Autodesk Inventor part; units mm, degrees
ref_plane "YZ Plane" through (0, 0, 0) normal (1, 0, 0) x (0, 1, 0)
ref_plane "XZ Plane" through (0, 0, 0) normal (0, 1, 0) x (-1, 0, 0)
ref_plane "XY Plane" through (0, 0, 0) normal (0, 0, 1) x (1, 0, 0)
sketch "Skizze1" plane through (0, 0, 0) normal (0, 1, 0) x (-1, 0, 0)
  line L0 (-37, 40) -> (37, 40)
  line L1 (40, 37) -> (40, -37)
  line L2 (37, -40) -> (-37, -40)
  line L3 (-40, -37) -> (-40, 37)
  line L4 (-40, 40) -> (40, -40) construction
  line L5 (40, 40) -> (-40, -40) construction
  arc A0 (40, 37) -> (37, 40) centre (37, 37) ccw
  arc A1 (-37, 40) -> (-40, 37) centre (-37, 37) ccw
  arc A2 (-40, -37) -> (-37, -40) centre (-37, -37) ccw
  arc A3 (37, -40) -> (40, -37) centre (37, -37) ccw
  point P0 (0, 0)
  dimension "d0" = 80
  dimension "d1" = 80
  dimension "d2" = 3
  dimension "d3" = 3
  dimension "d4" = 3
  dimension "d5" = 3
extrude "Extrusion1" add sketch "Skizze1" along normal blind 12
sketch "Skizze2" plane through (0, 12, 0) normal (0, 1, 0) x (1, 0, 0)
  line L0 (-40, 37) -> (-40, -37)
  arc A0 (-40, -37) -> (-37, -40) centre (-37, -37) ccw
  line L1 (-37, -40) -> (37, -40)
  arc A1 (37, -40) -> (40, -37) centre (37, -37) ccw
  line L2 (40, -37) -> (40, 37)
  arc A2 (40, 37) -> (37, 40) centre (37, 37) ccw
  line L3 (37, 40) -> (-37, 40)
  arc A3 (-37, 40) -> (-40, 37) centre (-37, 37) ccw
  line L4 (-35, -35) -> (-35, 35) construction
  line L5 (-35, 35) -> (35, 35) construction
  line L6 (35, 35) -> (35, -28)
  line L7 (28, -35) -> (-35, -35)
  line L8 (-35, -35) -> (-40, -35)
  line L9 (35, 35) -> (35, 40)
  arc A4 (28, -35) -> (35, -28) centre (32, -32) ccw
  point P0 (0, 0)
  dimension "d8" = 5
  dimension "d21" = 10
extrude "Extrusion2" cut sketch "Skizze2" against normal blind 6 contours A3 L3 L9 L6 A4 L7 L8 L0
fillet "Rundung1" radius 2 1 edges at (-40, 9, 35)
sketch "Skizze3" plane through (0, 0, 0) normal (0, -1, 0) x (1, 0, 0)
  arc A0 (-40, -37) -> (-37, -40) centre (-37, -37) ccw
  line L0 (-37, -37) -> (0, 0) construction
  line L1 (-37, -37) -> (-29.9289, -29.9289) construction
  dimension "d13" = 10
hole "Bohrung1" at (-29.9289, 0, -29.9289) direction (0, 1, 0) diameter 2.459 end through all
sketch "Skizze4" plane through (-37, 0, 40) normal (0, 0, 1) x (1, 0, 0)
  line L0 (-3, 0) -> (0, 0)
  line L1 (74, 0) -> (0, 0)
  line L2 (74, 0) -> (77, 0)
  line L3 (-3, 2) -> (0, 2)
  line L4 (0, 2) -> (74, 2)
  line L5 (74, 2) -> (77, 2)
  line L6 (-3, 0) -> (-3, 6)
  line L7 (77, 0) -> (77, 12)
  point P0 (37, 0)
  dimension "d22" = 2
extrude "Extrusion3" cut sketch "Skizze4" against normal blind 80
properties part number "Tastplatte" material "Aluminium 6061"
Geometry: final body of the model. Coordinates: model frame, mm. A direction names the side the tool comes from. Round coordinates to 2 decimals unless told otherwise and drop trailing zeros. Order: outer loops, then holes, each group sorted by start corner. A loop starts at its lowest first (then second) coordinate and runs counter-clockwise, first axis right, second up. Notation, with made-up numbers: (44, 63.25) - (91, 63.25) arc R4 cw to (91, 70.25) - close; hole circle Ø7 at (-10, 23.25). An arc over 180 degrees is marked (long way). Write item = value, one per line. Start each with the question number.
Q1. Access query for faces 5 (the cylindrical face through (39.14, 6.93, 39.1)), 6 (the cylindrical face through (-39.43, 8.96, 35.6)). Directions: +Z, -Z, +X, -X, +Y, -Y. A direction counts if a zero-diameter tool reaches every point of the face in a straight line with its end or side. Return the directions, or none.
Q2. Cut plane C-C on x = 32. Return the cut outline in (y, z), and give its area (3 significant figures).
Q3. Cut plane B-B on z = 7.5. Return the cut outline in (x, y).
Q4. Pull-direction query (X, two-part tool) for faces 1 (the flat face through (-5, 9, 35)), 2 (the cylindrical face through (-30.966, 4.028, -30.59)), 3 (the flat face through (-40, 4, 1)), 4 (the cylindrical face through (35, 9, 36)); classes: +X half, -X half, draft (parallel to the pull), parting line (faces both ways), or undercut.
Q5. Pin query (flat end, axial travel): pin 1 (4 mm diameter, centred on x = -9, z = -12, fed in from +Y); pin 2 (2 mm diameter, centred on y = 10.5, z = 18.5, fed in from -X); pin 3 (2 mm diameter, centred on x = -29.93, z = -29.93, fed in from +Y). Return the tip coordinate at first contact, or that it passes through.
Q6. Ray query, line 1 (Y direction, x = 23.5, z = 33.5); line 2 (Z direction, x = 5, y = 10.25). Return the intervals inside material, ascending. Write a range as from..to.
Outcome:
q1.face_5 = +Z, +X, +Y, -Y
q1.face_6 = -Z, -X, +Y
q2.outline = (2, -40) - (6, -40) - (6, 37) - (12, 37) - (12, 40) - (2, 40) - close
q2.area = 338 mm^2
q3.outline = (-40, 2) - (40, 2) - (40, 12) - (35, 12) - (35, 6) - (-40, 6) - close
q4.face_1 = draft
q4.face_2 = undercut
q4.face_3 = -X half
q4.face_4 = undercut
q5.pin_1 = 6
q5.pin_2 = 35
q5.pin_3 = through
q6.line_1 = 2..6
q6.line_2 = 35..40
